Autodesk Inventor part; units mm, degrees
ref_plane "YZ Plane" through (0, 0, 0) normal (1, 0, 0) x (0, 1, 0)
ref_plane "XZ Plane" through (0, 0, 0) normal (0, 1, 0) x (-1, 0, 0)
ref_plane "XY Plane" through (0, 0, 0) normal (0, 0, 1) x (1, 0, 0)
sketch "Sketch1" plane through (0, 0, 0) normal (1, 0, 0) x (0, 1, 0)
  line L0 (0, 0) -> (0, 194.818) construction
  line L1 (20.32, 0) -> (20.32, 194.818)
  line L2 (-20.32, 194.818) -> (-20.32, 0)
  arc A0 (-20.32, 0) -> (20.32, 0) centre (0, 0) ccw
  arc A1 (20.32, 194.818) -> (-20.32, 194.818) centre (0, 194.818) ccw
  line L3 (23.495, 194.818) -> (23.495, 0)
  arc A2 (-23.495, 0) -> (23.495, 0) centre (0, 0) ccw
  line L4 (-23.495, 0) -> (-23.495, 194.818)
  arc A3 (23.495, 194.818) -> (-23.495, 194.818) centre (0, 194.818) ccw
  point P0 (0, 97.409)
  dimension "d0" = 194.818
  dimension "d1" = 40.64
  dimension "d2" = 3.175
extrude "Extrusion1" add sketch "Sketch1" along normal blind 127
properties part number "Shooting_Belt"
Geometry: final body of the model. Coordinates: model frame, mm. A direction names the side the tool comes from. Give positions to 0.01 mm unless a question says otherwise; leave off trailing zeros. Order: outer loops, then holes, each group sorted by start corner. A loop starts at its lowest first (then second) coordinate and runs counter-clockwise, first axis right, second up. Notation, with made-up numbers: (83, -2) -> (129, -2) arc R33 cw to (129, 26) -> close; hole circle Ø5 at (-25, -29). An arc over 180 degrees is marked (long way). Put each result on its own line as item: value.
Q1. Pin query (flat end, axial travel): pin 1 (3 mm diameter, centred on x = 80.5, y = -12, fed in from +Z); pin 2 (2 mm diameter, centred on x = 56, y = 7.5, fed in from +Z). Return the tip coordinate at first contact, or that it passes through.
Here are the results:
pin 1: stops at z = 215.84
pin 2: stops at z = 217.4
Q2. Section B-B, the plane y = 0. Return loops of the section in (x, z) (3 decimals), then the cut area to 3 significant figures.
Here are the results:
outline: (0, -23.495) -> (127, -23.495) -> (127, -20.32) -> (0, -20.32) -> close; (0, 215.138) -> (127, 215.138) -> (127, 218.313) -> (0, 218.313) -> close
area: 806 mm^2
Q3. Draft query along Z for faces 3 (the face through (62.61, 0.52, -23.49)), 4 (the face through (63, -23.495, 96)), 5 (the face through (62.611, 0.447, -20.315)), 6 (the face through (62.611, -0.517, 218.307)). Return one class per face: released by +Z, released by -Z, zero draft, split by the parting line, or undercut.
Here are the results:
face 3: released by -Z
face 4: zero draft
face 5: undercut
face 6: released by +Z
Q4. Reachability of faces 1 (the face through (127, 21, 98)), 2 (the face through (62.611, -0.447, 215.133)) from +Z, -Z, +X, -X, +Y, -Y: full face, straight path, thin tool, end or side. Return the list, or none.
Here are the results:
face 1: +Z, -Z, +X, +Y, -Y
face 2: +X, -X
Q5. Section A-A, the plane x = 111.5. Return loops of the section in (y, z) (3 decimals), then the cut area to 3 significant figures.
Here are the results:
outline: (-23.495, 0) arc R23.495 ccw to (23.495, 0) -> (23.495, 194.818) arc R23.495 ccw to (-23.495, 194.818) -> close; hole (-20.32, 0) arc R20.32 ccw to (20.32, 0) -> (20.32, 194.818) arc R20.32 ccw to (-20.32, 194.818) -> close
area: 1,670 mm^2
Q6. Section C-C, the plane z = 181. Return loops of the section in (x, y) (3 decimals).
Here are the results:
outline: (0, -23.495) -> (127, -23.495) -> (127, -20.32) -> (0, -20.32) -> close; (0, 20.32) -> (127, 20.32) -> (127, 23.495) -> (0, 23.495) -> close
Q7. Material intervals for L1, parallel to Y at x = 46, z = 36 (3 decimals); L2, parallel to Z at x = 88, y = 0 (3 decimals); L3, parallel to Y at x = 19.5, z = 201, sorted ascending.
Here are the results:
L1: y = -23.495 to -20.32, 20.32 to 23.495
L2: z = -23.495 to -20.32, 215.138 to 218.313
L3: y = -22.67 to -19.36, 19.36 to 22.67
